Could you check a few things on this model? Use its own coordinates, in mm. Round coordinates to 2 decimals unless told otherwise and drop trailing zeros. Loops run counter-clockwise (first coordinate to the right, second up) from the corner with the lowest first, then second, coordinate; pieces in that order, holes last. Notation, with made-up numbers: M -38.75,2 L 16.25,2 A15 cw 16.25,16 Z; hole C -1,86 d2. An arc over 180 degrees is marked long. Answer in a Markdown table with one row per item.
```python
from build123d import *

# Parameters (mm, degrees)
F1_DEPTH = 10
F1_TAPER = 3


with BuildPart() as f1:
    # F0 (on Top) → F1 (new body)
    with BuildSketch(Plane.XY):
        Polygon((3, -1.7320508076), (3, 1.7320508076), (0, 3.4641016151), (-3, 1.7320508076), (-3, -1.7320508076), (0, -3.4641016151), align=None)
    extrude(amount=F1_DEPTH, taper=F1_TAPER)


with BuildPart() as f4:
    # F3 (on 3pt) → F4 (revolve)
    with BuildSketch(Plane(origin=(0, 0, 0), x_dir=(0.8660254038, -0.5, 0), z_dir=(-0.5, -0.8660254038, 0))):
        with BuildLine():
            Line((0, 0), (0, 0.2533346897))
            ThreePointArc((0, 0.2533346897), (-1.7412651517, 0.2526643975), (-3.4641016151, 0))
            Line((-3.4641016151, 0), (0, 0))
        make_face()
    revolve(axis=Axis((0, 0, 0.1266673449), (0, 0, -1)))


with BuildPart() as f1_1:
    add(f1.part)

    # F5: cut F4
    add(f4.part, mode=Mode.SUBTRACT)


solid = f1_1.part
```
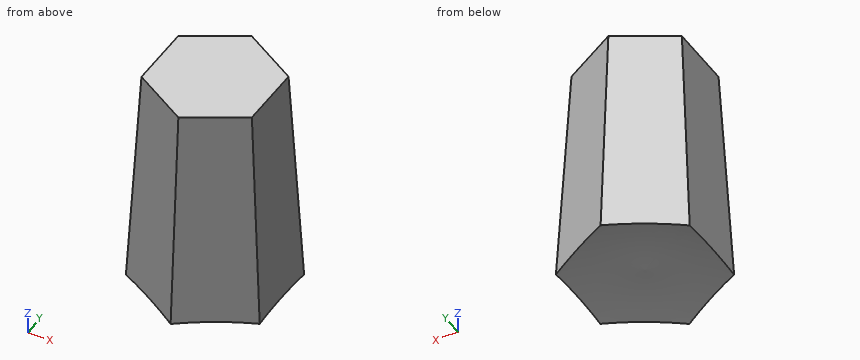
1) I want a section at B-B, the plane z = 5.5. Please give me the cut outline in (x, y).
Computed:
| item | result |
|---|---|
| outline | M -2.71,-1.57 L 0,-3.13 L 2.71,-1.57 L 2.71,1.57 L 0,3.13 L -2.71,1.57 Z |
2) Will these pins go through, and if not, where does the flat tip stop? P1, Ø1.5, axis at y = -2, z = 8.5, coming from the +X side; P2, Ø3, axis at y = 1, z = 4, coming from the -X side; P3, Ø1, axis at y = -2.5, z = 4, coming from the +X side.
Computed:
| item | result |
|---|---|
| P1 | stops at x = 2.58 |
| P2 | stops at x = -2.87 |
| P3 | stops at x = 2.12 |
3) I need wall thicknesses on line 1 (Z direction, x = -1, y = 0.25); line 2 (X direction, y = -1.75, z = 6.5); line 3 (Y direction, x = 2, z = 5.25). Which ranges of each line are inside material? Lowest first, please.
Computed:
| item | result |
|---|---|
| line 1 | z = 0.28 to 10 |
| line 2 | x = -2.29 to 2.29 |
| line 3 | y = -1.99 to 1.99 |
4) I want a section at A-A, the plane z = 4. Please give me the cut outline in (x, y).
Computed:
| item | result |
|---|---|
| outline | M -2.79,-1.61 L 0,-3.22 L 2.79,-1.61 L 2.79,1.61 L 0,3.22 L -2.79,1.61 Z |
